```python
from build123d import *

# Parameters (mm, degrees)
CHAMFER1_SIZE  = 1
CHAMFER2_SIZE  = 0.5
EXTRUDE2_DEPTH = 10
CHAMFER3_SIZE  = 0.5
CHAMFER4_SIZE  = 0.2


with BuildPart() as part:
    # Sketch1 → Revolve1 (revolve)
    with BuildSketch(Plane.XY, mode=Mode.PRIVATE) as revolve1_sk:
        Polygon((0, 0), (0, 5.9), (-2.5, 5.9), (-2.5, 10), (-17.5, 10), (-17.5, 9), (-19.5, 9), (-19.5, 15), (-24.5, 15), (-24.5, 13), (-21, 13), (-21, 0), align=None)
    revolve(revolve1_sk.sketch.rotate(Axis((-24.5, 0, 0), (1, 0, 0)), 90), axis=Axis((-24.5, 0, 0), (1, 0, 0)))

    # Chamfer1
    chamfer1_edges = [part.edges().sort_by_distance(p)[0] for p in [
        (-2.5, 0, -10),
    ]]
    chamfer(chamfer1_edges, length=CHAMFER1_SIZE)

    # Chamfer2
    chamfer2_edges = [part.edges().sort_by_distance(p)[0] for p in [
        (0, 0, -5.9),
    ]]
    chamfer(chamfer2_edges, length=CHAMFER2_SIZE)

    # Sketch2 → Extrude2 (cut)
    with BuildSketch(Plane.ZY.offset(21)):
        with BuildLine():
            ThreePointArc((9.578114368, 5.40922593), (10.601186453, 5.129330555), (10.881081828, 6.152402641))
            ThreePointArc((10.881081828, 6.152402641), (0.026245134, 12.499972448), (-10.855150648, 6.198040369))
            ThreePointArc((-10.855150648, 6.198040369), (-10.859121552, 6.19108061), (-10.863087994, 6.184118308))
            ThreePointArc((-10.863087994, 6.184118308), (-10.579057999, 5.168029786), (-9.559993103, 5.441188461))
            ThreePointArc((-9.559993103, 5.441188461), (0.018371062, 10.999984659), (9.578114368, 5.40922593))
        make_face()
    extrude(amount=-EXTRUDE2_DEPTH, mode=Mode.SUBTRACT)

    # Chamfer3
    chamfer3_edges = [part.edges().sort_by_distance(p)[0] for p in [
        (-19.5, 0, -15),
        (-24.5, 0, -15),
    ]]
    chamfer(chamfer3_edges, length=CHAMFER3_SIZE)

    # Chamfer4
    chamfer4_edges = [part.edges().sort_by_distance(p)[0] for p in [
        (-24.5, 0, -13),
    ]]
    chamfer(chamfer4_edges, length=CHAMFER4_SIZE)


solid = part.part
```
Geometry check sheet. Reference: the model listing, model coordinates, mm. A direction names the side the tool comes from. Coordinates: 2 decimals unless noted, no trailing zeros. Write each loop counter-clockwise with the first axis right and the second up, starting at its lowest first coordinate (ties: lowest second). Pieces come first, ordered by that corner, then holes. Notation, with made-up numbers: M 19,48 L 44,48 A12 cw 44,54 Z; hole C 46,61.25 d11. An arc over 180 degrees is marked long. Answer as a JSON object with one key per item and string values.
1. Section check C-C, the plane x = -7.5. Enter the section's corners in (y, z), plus the area to 3 significant figures.
Answers below:
{"outline": "C 0,0 d20", "area": "314 mm²"}
2. Go/stop test with flat-tipped pins: pin 1 Ø4 at (x, y) = (-13, -8) entering from +Z; pin 2 Ø5.5 at (y, z) = (-2, 1) entering from +X; pin 3 Ø8 at (y, z) = (-9, 7) entering from +X; pin 4 Ø1 at (x, z) = (-17.5, 5) entering from +Y. Record where each tip stops, or that it passes through.
Answers below:
{"pin 1": "stops at z = 8", "pin 2": "stops at x = 0", "pin 3": "stops at x = -2.5", "pin 4": "stops at y = 8.93"}
3. Scan lines: L1, parallel to Y at x = -22.95, z = 0; L2, parallel to X at y = 2.5, z = -10; L3, parallel to Y at x = -22, z = -6.75. Record each from-to range of solid material in increasing order.
Answers below:
{"L1": "y = -15 to -13, 13 to 15", "L2": "x = -21 to -19.5", "L3": "y = -13.4 to -11.11, 11.11 to 13.4"}
4. Tool access check on faces 1 (the cylindrical face through (-22.627, 7.91, -10.316)), 2 (the cylindrical face through (-11, 0, -10)), 3 (the cylindrical face through (-20, 11, 0)), 4 (the flat face through (-19.5, -7, -6)). Record the directions out of +Z, -Z, +X, -X, +Y, -Y that give a thin tool (end or side, any length) a straight path to the whole face; none if there is none.
Answers below:
{"face 1": "-X", "face 2": "+X", "face 3": "+X, -X", "face 4": "none"}
5. Draft check along Y on faces 5 (the cylindrical face through (-1.514, -0.259, -5.894)), 6 (the flat face through (-24.5, 12, 6)), 7 (the flat face through (-21, 0, 0)). Enter one of: released by +Y, released by -Y, zero draft, split by the parting line, or undercut.
Answers below:
{"face 5": "split by the parting line", "face 6": "zero draft", "face 7": "undercut"}
